```python
from build123d import *

# Parameters (mm, degrees)
SKETCH1_R           = 2.25
BOSS_EXTRUDE1_DEPTH = 19.05
SKETCH2_W           = 23.025
SKETCH2_H           = 6.858
CUT_EXTRUDE1_DEPTH  = 19.05


with BuildPart() as part:
    # Sketch1 → Boss-Extrude1 (new body)
    with BuildSketch(Plane(origin=(0, 0, 0), x_dir=(1, 0, 0), z_dir=(0, 1, 0))):
        with BuildLine():
            Line((0, 6), (100, 6))
            ThreePointArc((100, 6), (106, 0), (100, -6))
            Line((100, -6), (0, -6))
            ThreePointArc((0, -6), (-6, 0), (0, 6))
        make_face()
        with Locations(Location((0, 0, 0), (0, 0, 90))):
            Circle(SKETCH1_R, mode=Mode.SUBTRACT)
        with Locations(Location((100, 0, 0), (0, 0, 90))):
            Circle(SKETCH1_R, mode=Mode.SUBTRACT)
    extrude(amount=BOSS_EXTRUDE1_DEPTH)

    # Sketch2 → Cut-Extrude1 (cut)
    with BuildSketch(Plane(origin=(0, 0, -6), x_dir=(-1, 0, 0), z_dir=(0, 0, -1))):
        with Locations((1.9875, 9.525)):
            Rectangle(SKETCH2_W, SKETCH2_H)
    cut_extrude1 = extrude(amount=-CUT_EXTRUDE1_DEPTH, mode=Mode.SUBTRACT)

    # Mirror1: Cut-Extrude1 across plane
    add(cut_extrude1.mirror(Plane(origin=(50, 0, 0), x_dir=(0, 0, 1), z_dir=(1, 0, 0))), mode=Mode.SUBTRACT)


solid = part.part
```
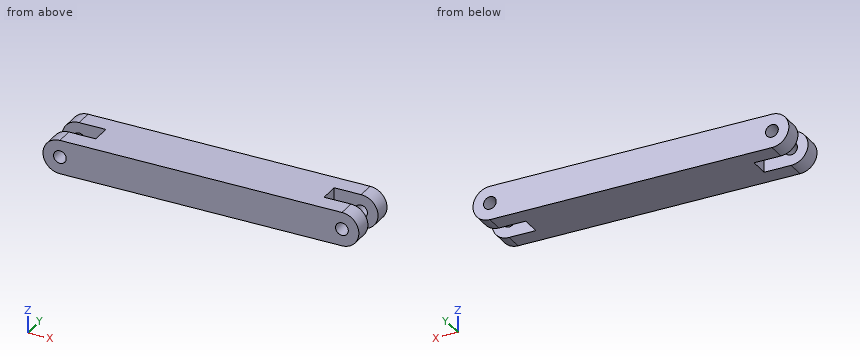
Source: CAD feature listing. Evaluate the final solid. Frame: model axes, mm. Give positions to 0.01 mm unless a question says otherwise; leave off trailing zeros. Loops run counter-clockwise (first coordinate to the right, second up) from the corner with the lowest first, then second, coordinate; pieces in that order, holes last. Notation, with made-up numbers: (40.25, 70.25) - (78.25, 70.25) arc R13 ccw to (78.25, 74.25) - close; hole circle Ø5 at (-9.75, 33.25). An arc over 180 degrees is marked (long way). Use CSV: the item, a comma, the result in double quotes.
1) Cut plane C-C (z = 0). Output: boundary loops of the cut face in (x, y) (3 decimals), and give its area (3 significant figures).
Worked out:
outline,"(-6, 0) - (-2.25, 0) - (-2.25, 6.096) - (-6, 6.096) - close; (-6, 12.954) - (-2.25, 12.954) - (-2.25, 19.05) - (-6, 19.05) - close; (2.25, 0) - (97.75, 0) - (97.75, 6.096) - (90.475, 6.096) - (90.475, 12.954) - (97.75, 12.954) - (97.75, 19.05) - (2.25, 19.05) - (2.25, 12.954) - (9.525, 12.954) - (9.525, 6.096) - (2.25, 6.096) - close; (102.25, 0) - (106, 0) - (106, 6.096) - (102.25, 6.096) - close; (102.25, 12.954) - (106, 12.954) - (106, 19.05) - (102.25, 19.05) - close"
area,"1,810 mm^2"
2) Line query: line 1 (X direction, y = 3.25, z = 0); line 2 (Z direction, x = 100, y = 3); line 3 (Y direction, x = -1, z = -4). Output: solid intervals per line, ascending.
Worked out:
line 1,"x = -6 to -2.25, 2.25 to 97.75, 102.25 to 106"
line 2,"z = -6 to -2.25, 2.25 to 6"
line 3,"y = 0 to 6.1, 12.95 to 19.05"
3) Pin query (flat end, axial travel): P1, Ø7, axis at x = 100, z = 0, coming from the +Y side; P2, Ø1, axis at y = 12, z = 2.5, coming from the +X side (3 decimals); P3, Ø5.5, axis at y = 8.5, z = 1.5, coming from the +X side. Return the tip coordinate at first contact, or that it passes through.
Worked out:
P1,"stops at y = 19.05"
P2,"stops at x = 90.475"
P3,"stops at x = 106"
4) Cut plane B-B (y = 1.5). Output: boundary loops of the cut face in (x, z), and give its area (3 significant figures).
Worked out:
outline,"(0, -6) - (100, -6) arc R6 ccw to (100, 6) - (0, 6) arc R6 ccw to start; hole circle Ø4.5 at (0, 0); hole circle Ø4.5 at (100, 0)"
area,"1,280 mm^2"
5) Cut plane A-A (x = 5). Output: boundary loops of the cut face in (y, z), and give its area (3 significant figures).
Worked out:
outline,"(0, -6) - (6.1, -6) - (6.1, 6) - (0, 6) - close; (12.95, -6) - (19.05, -6) - (19.05, 6) - (12.95, 6) - close"
area,"146 mm^2"
6) Cut plane D-D (y = 11.5). Output: boundary loops of the cut face in (x, z) (3 decimals).
Worked out:
outline,"(9.525, -6) - (90.475, -6) - (90.475, 6) - (9.525, 6) - close"
